```python
from build123d import *

# Parameters (mm, degrees)
SKETCH1_R           = 52.3875
SKETCH1_R_2         = 49.2125
BOSS_EXTRUDE1_DEPTH = 38.1
SKETCH2_R           = 50.8
SKETCH2_R_2         = 49.2125
BOSS_EXTRUDE2_DEPTH = 9.525
SKETCH3_R           = 57.15
SKETCH3_R_2         = 52.3875
BOSS_EXTRUDE3_DEPTH = 3.175


with BuildPart() as part:
    # Sketch1 → Boss-Extrude1 (new body)
    with BuildSketch(Plane(origin=(0, 0, 0), x_dir=(1, 0, 0), z_dir=(0, 1, 0))):
        Circle(SKETCH1_R)
        Circle(SKETCH1_R_2, mode=Mode.SUBTRACT)
    extrude(amount=BOSS_EXTRUDE1_DEPTH)

    # Sketch2 → Boss-Extrude2 (add)
    with BuildSketch(Plane.XZ):
        Circle(SKETCH2_R)
        Circle(SKETCH2_R_2, mode=Mode.SUBTRACT)
    extrude(amount=BOSS_EXTRUDE2_DEPTH)

    # Sketch3 → Boss-Extrude3 (add)
    with BuildSketch(Plane.XZ):
        Circle(SKETCH3_R)
        Circle(SKETCH3_R_2, mode=Mode.SUBTRACT)
    extrude(amount=-BOSS_EXTRUDE3_DEPTH)


solid = part.part
```
Input: part model. Units: mm. Frame: model coordinates. A direction names the side the tool comes from. Round coordinates to 2 decimals unless told otherwise and drop trailing zeros. Write each loop counter-clockwise with the first axis right and the second up, starting at its lowest first coordinate (ties: lowest second). Pieces come first, ordered by that corner, then holes. Notation, with made-up numbers: M 1.5,11 L 24.5,11 A17 cw 24.5,32 Z; hole C 40,31 d3. An arc over 180 degrees is marked long. Write each question's results on one line, items separated by ' | '.
Q1. Line query: line 1 along Z through (x, y) = (0, 8); line 2 along Z through (x, y) = (-8, -6). Output: solid intervals per line, ascending.
Results:
line 1: z = -52.39 to -49.21, 49.21 to 52.39 | line 2: z = -50.17 to -48.56, 48.56 to 50.17
Q2. Section query C-C (y = 18). Return loops of the section in (x, z) (1 decimal), and give its area (3 significant figures).
Results:
outline: C 0,0 d104.8; hole C 0,0 d98.4 | area: 1,010 mm^2
Q3. Pin query (flat end, axial travel): P1, Ø1, axis at y = 31, z = 6.5, coming from the +X side; P2, Ø1.5, axis at y = 32, z = -26, coming from the -X side; P3, Ø10, axis at y = 23.5, z = 27.5, coming from the -X side. Return the tip coordinate at first contact, or that it passes through.
Results:
P1: stops at x = 52.04 | P2: stops at x = -45.9 | P3: stops at x = -47.31
Q4. Access query for faces 1 (the face through (-11.012, -4.696, -49.592)), 2 (the face through (-11.36, 20.39, 51.14)), 3 (the face through (-42, -9.525, 27)). Directions: +Z, -Z, +X, -X, +Y, -Y. A direction counts if a zero-diameter tool reaches every point of the face in a straight line with its end or side. Return the directions, or none.
Results:
face 1: -Y | face 2: +Y | face 3: +Z, -Z, +X, -X, -Y
